from build123d import *

# Parameters (mm, degrees)
SKETCH_1_W          = 30
SKETCH_1_H          = 30
SKETCH_1_R          = 5
EXTRUDE_1_DEPTH     = 15
SKETCH_3_R          = 8
CUT_EXTRUDE_1_DEPTH = 5


with BuildPart() as part:
    # 草圖1 → 填料-伸長1 (new, symmetric)
    with BuildSketch(Plane.XY):
        with Locations((15, 15)):
            Rectangle(SKETCH_1_W, SKETCH_1_H)
        with Locations((15, 15)):
            Circle(SKETCH_1_R, mode=Mode.SUBTRACT)
    extrude(amount=EXTRUDE_1_DEPTH, both=True)

    # 草圖3 → 除料-伸長1 (cut)
    with BuildSketch(Plane.XY.offset(15)):
        with Locations((15, 15)):
            Circle(SKETCH_3_R)
    cut_extrude_1 = extrude(amount=-CUT_EXTRUDE_1_DEPTH, mode=Mode.SUBTRACT)

    # 鏡射1: 除料-伸長1 across plane
    add(cut_extrude_1.mirror(Plane.XY), mode=Mode.SUBTRACT)


solid = part.part
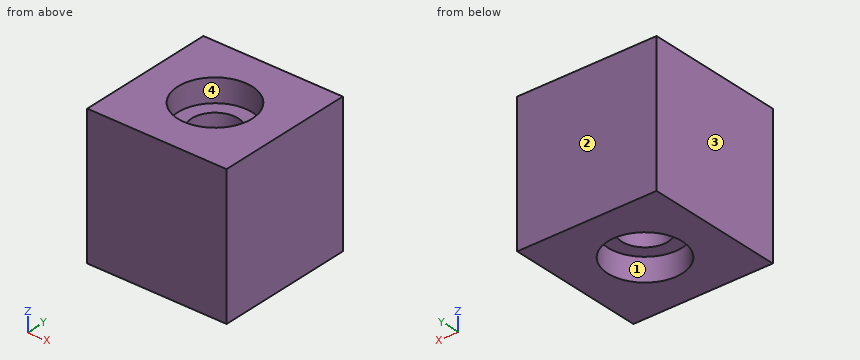
The model under review builds one solid part; all positions refer to its coordinate system, in mm. Face numbers are marked on the shaded views. Coordinates: 2 decimals unless noted, no trailing zeros. Loops run counter-clockwise (first coordinate to the right, second up) from the corner with the lowest first, then second, coordinate; pieces in that order, holes last. Notation, with made-up numbers: M 21.5,-31 L 26.5,-31 A11 ccw 26.5,-23 Z; hole C 29.5,-10.5 d8. An arc over 180 degrees is marked long. Put each result on its own line as item: value. Start each with the question number.
Q1. Add section C-C (z = -12). Write out the cut boundary in (x, y), and give its area (3 significant figures).
Q2. Clearance check with flat-ended pins moving along their axes: pin 1 (11.5 mm diameter, centred on x = 15, y = 15, fed in from +Z); pin 2 (8 mm diameter, centred on x = 16.5, y = 14.5, fed in from -Z). State where each tip first meets the part, or that it passes through.
Q3. Add section A-A (x = 15). Write out the cut boundary in (y, z), and give its area (3 significant figures).
Q4. Add section D-D (z = 5.5). Write out the cut boundary in (x, y), and give its area (3 significant figures).
Q5. Wall thickness on line 1 (Y direction, x = 15, z = 12.5); line 2 (Y direction, x = 15, z = -1.25); line 3 (X direction, y = 14, z = 6.5): over which ranges is each line inside the solid? List them lowest first.
Q6. The part is to be moulded in two halves that separate along X. For the marked faces 1, 2, 3 and 4, say which applies: +X half, -X half, draft (parallel to the pull), parting line (faces both ways), or undercut.
Answers:
1. outline: M 0,0 L 30,0 L 30,30 L 0,30 Z; hole C 15,15 d16
1. area: 699 mm^2
2. pin 1: stops at z = 10
2. pin 2: stops at z = -10
3. outline: M 0,-15 L 7,-15 L 7,-10 L 10,-10 L 10,10 L 7,10 L 7,15 L 0,15 Z; M 20,-10 L 23,-10 L 23,-15 L 30,-15 L 30,15 L 23,15 L 23,10 L 20,10 Z
3. area: 540 mm^2
4. outline: M 0,0 L 30,0 L 30,30 L 0,30 Z; hole C 15,15 d10
4. area: 821 mm^2
5. line 1: y = 0 to 7, 23 to 30
5. line 2: y = 0 to 10, 20 to 30
5. line 3: x = 0 to 10.1, 19.9 to 30
6. face 1: undercut
6. face 2: draft
6. face 3: -X half
6. face 4: undercut
